from build123d import *

# Parameters (mm, degrees)
PAD015_DEPTH    = 46.5
SKETCH024_R     = 3.175
POCKET016_DEPTH = 4
FILLET007_R     = 4


with BuildPart() as part:
    # Sketch043 → Pad015 (new body, symmetric)
    with BuildSketch(Plane.YZ):
        Polygon((-268, 55), (-268.9285051775, 57.8526966427), (-175.7404148487, 88.1838657739), (-61.2329665245, 57.900286132), (-62, 55), (-175.5643554306, 85.0341615546), align=None)
    extrude(amount=PAD015_DEPTH, both=True)

    # Sketch024 (on Face2 of Pad015) → Pocket016 (cut)
    with BuildSketch(Plane(origin=(0, -42.7873449396, 131.4578725241), x_dir=(0, -0.9508988809, -0.3095017258), z_dir=(0, -0.3095017258, 0.9508988809))):
        with Locations((157.8183051623, -31)):
            Circle(SKETCH024_R)
        with Locations((157.8183051623, 31)):
            Circle(SKETCH024_R)
        with Locations((219.8183051623, 31)):
            Circle(SKETCH024_R)
        with Locations((219.8183051623, -31)):
            Circle(SKETCH024_R)
    extrude(amount=-POCKET016_DEPTH, mode=Mode.SUBTRACT)

    # Fillet007
    fillet007_edges = [part.edges().sort_by_distance(p)[0] for p in [
        (0, -175.740415, 88.183866),
        (0, -175.564355, 85.034162),
    ]]
    fillet(fillet007_edges, radius=FILLET007_R)


with BuildPart() as part_1:
    # Body009 placement: moved
    add(part.part.moved(Location((0, 0, 1))))


solid = part_1.part
Geometry: final body of the model. Coordinates: model frame, mm. A direction names the side the tool comes from. Coordinates: 2 decimals unless noted, no trailing zeros. Loops run counter-clockwise (first coordinate to the right, second up) from the corner with the lowest first, then second, coordinate; pieces in that order, holes last. Notation, with made-up numbers: (-25.75, 2.25) - (-13.75, 2.25) arc R19 cw to (-13.75, 33.25) - close; hole circle Ø11 at (62.25, 42). An arc over 180 degrees is marked (long way). One line per question, with ' | ' between items. Start each with the question number.
(1) Draft query along Y for faces 1 (the cylindrical face through (-32.932, -248.957, 63.792)), 2 (the flat face through (0.651, -223.539, 73.626)), 3 (the flat face through (46.5, -165, 84)), 4 (the flat face through (0.7, -118.7, 74.1)). Return one class per face: +Y half, -Y half, draft (parallel to the pull), parting line (faces both ways), or undercut.
(2) Cut plane B-B on z = 77.5. Output: boundary loops of the cut face in (x, y), and give its area (3 significant figures).
(3) Reachability of faces 5 (the flat face through (0.65, -117.43, 70.66)), 6 (the cylindrical face through (-32.22, -195.18, 81.28)) from +Z, -Z, +X, -X, +Y, -Y: full face, straight path, thin tool, end or side. Return the list, or none.
(4) Cut plane D-D on y = -170.5. Output: boundary loops of the cut face in (x, z), and give its area (3 significant figures).
(5) Ray query, L1, parallel to Z at x = -33, y = -237; L2, parallel to Z at x = 23, y = -177.5. Return the intervals inside material, ascending. Write a range as from..to.
(6) Cut plane A-A on x = 18.5. Output: boundary loops of the cut face in (y, z).
(7) First-contact query: pin 1 (8 mm diameter, centred on x = 17.5, y = -119, fed in from -Z); pin 2 (2 mm diameter, centred on x = -9, y = -188, fed in from +Z); pin 3 (1 mm diameter, centred on x = 30, y = -182, fed in from -Z). Flat tips, straight axial feed; report the tip coordinate or a pass-through.
(8) Cut plane C-C on y = -222.5. Output: boundary loops of the cut face in (x, z).
Here are the results:
1) face 1: undercut | face 2: -Y half | face 3: draft | face 4: +Y half
2) outline: (-46.5, -211.64) - (46.5, -211.64) - (46.5, -201.83) - (-46.5, -201.83) - close; (-46.5, -143.3) - (46.5, -143.3) - (46.5, -131.56) - (-46.5, -131.56) - close | area: 2,000 mm²
3) face 5: -Z, +X, -X | face 6: none
4) outline: (-46.5, 84.69) - (46.5, 84.69) - (46.5, 87.8) - (-46.5, 87.8) - close | area: 289 mm²
5) L1: 66.07..69.24 | L2: 85.41..88.61
6) outline: (-268.93, 58.85) - (-268, 56) - (-176.68, 85.67) arc R4 cw to (-174.43, 85.73) - (-62, 56) - (-61.23, 58.9) - (-174.6, 88.88) arc R4 ccw to (-176.86, 88.82) - close
7) pin 1: z = 70.02 | pin 2: z = 85.52 | pin 3: z = 83.78
8) outline: (-46.5, 70.78) - (46.5, 70.78) - (46.5, 73.96) - (-46.5, 73.96) - close
